The model under review builds one solid part; all positions refer to its coordinate system, in mm. A direction names the side the tool comes from. Round coordinates to 2 decimals unless told otherwise and drop trailing zeros. Loops run counter-clockwise (first coordinate to the right, second up) from the corner with the lowest first, then second, coordinate; pieces in that order, holes last. Notation, with made-up numbers: (40, -39.5) -> (70, -39.5) arc R12 cw to (70, -33.5) -> close; hole circle Ø7 at (58, 46). An arc over 180 degrees is marked (long way). Return JSON: item names as keys, results as strings. Group by question number.
```python
from build123d import *

# Parameters (mm, degrees)
SKETCH1_W           = 20.3
SKETCH1_H           = 20.5
BOSS_EXTRUDE1_DEPTH = 1.65
FILLET1_R           = 2
SKETCH2_R           = 1.25
CUT_EXTRUDE1_DEPTH  = 15.519211411
BOSS_EXTRUDE2_DEPTH = 2.65
SKETCH4_W           = 0.64
SKETCH4_H           = 0.64
BOSS_EXTRUDE3_DEPTH = 6
LPATTERN1_COUNT     = 7
LPATTERN1_PITCH     = 2.5
SKETCH5_W           = 17.5
SKETCH5_H           = 11
BOSS_EXTRUDE4_DEPTH = 1.35


with BuildPart() as part:
    # Sketch1 → Boss-Extrude1 (new body)
    with BuildSketch(Plane(origin=(0, 0, 0), x_dir=(1, 0, 0), z_dir=(0, 1, 0))):
        Rectangle(SKETCH1_W, SKETCH1_H)
    extrude(amount=BOSS_EXTRUDE1_DEPTH)

    # Fillet1
    fillet1_edges = [part.edges().sort_by_distance(p)[0] for p in [
        (10.15, 0.825, 10.25),
        (-10.15, 0.825, 10.25),
        (-10.15, 0.825, -10.25),
        (10.15, 0.825, -10.25),
    ]]
    fillet(fillet1_edges, radius=FILLET1_R)

    # Sketch2 → Cut-Extrude1 (cut, through all)
    with BuildSketch(Plane(origin=(0, 1.65, 0), x_dir=(1, 0, 0), z_dir=(0, 1, 0))):
        with Locations(Location((7.9, -8.1, 0), (0, 0, 270))):
            Circle(SKETCH2_R)
        with Locations(Location((-7.9, -8.1, 0), (0, 0, 270))):
            Circle(SKETCH2_R)
    extrude(amount=-CUT_EXTRUDE1_DEPTH, mode=Mode.SUBTRACT)

    # Sketch3 → Boss-Extrude2 (add)
    with BuildSketch(Plane(origin=(0, 1.65, 0), x_dir=(1, 0, 0), z_dir=(0, 1, 0))):
        Polygon((-8.395, 9.85), (-6.602128422, 9.85), (-6.248596673, 9.496424969), (-6.248596673, 7.703553391), (-6.602150064, 7.35), (-8.395021642, 7.35), (-8.748553391, 7.703575031), (-8.748553391, 9.496446609), align=None)
    boss_extrude2 = extrude(amount=BOSS_EXTRUDE2_DEPTH)

    # Sketch4 → Boss-Extrude3 (add)
    with BuildSketch(Plane(origin=(0, 4.3, 0), x_dir=(1, 0, 0), z_dir=(0, 1, 0))):
        with Locations((-7.498564211, 8.60001082)):
            Rectangle(SKETCH4_W, SKETCH4_H)
    boss_extrude3 = extrude(amount=BOSS_EXTRUDE3_DEPTH)

    # LPattern1: Boss-Extrude2, Boss-Extrude3 ×7
    with Locations(*[(i * LPATTERN1_PITCH, 0, 0) for i in range(1, LPATTERN1_COUNT)]):
        add(boss_extrude2)
        add(boss_extrude3)

    # Sketch5 → Boss-Extrude4 (add)
    with BuildSketch(Plane.XZ):
        with Locations((0, -1)):
            Rectangle(SKETCH5_W, SKETCH5_H)
    extrude(amount=BOSS_EXTRUDE4_DEPTH)


solid = part.part
```
1. For P1, Ø2, axis at y = 4, z = -7, coming from the +X side; P2, Ø0.7, axis at x = 5, y = 8, coming from the +Z side; P3, Ø0.5, axis at x = 5, y = 2.5, coming from the -Z side, all flat-tipped, find the tip position at first contact; note any pin that passes through.
2. We need section C-C, the plane y = 2.75. Give the number of separate pieces and of enclosed holes in the cut face, then the cut area to 3 significant figures.
3. Tool access review of faces 1 (the face through (3, 3, -7.35)), 2 (the face through (-8.749, 3, -9)), 3 (the face through (-3, 3, -9.85)), 4 (the face through (8.75, -1, -1)): name each direction out of +Z, -Z, +X, -X, +Y, -Y from which nothing blocks a thin tool from reaching the whole face with its end or side.
4. We need section A-A, the plane y = 7. Write out the cut boundary in (x, z).
5. We need section B-B, the plane z = -5. Write out the cut boundary in (x, y).
6. Wall thickness on line 1 (X direction, y = 1, z = 8.1); line 2 (Y direction, x = -2, z = -1.75); line 3 (Y direction, x = 9.25, z = 8): over which ranges is each line inside the solid? List them lowest first.
Check sheet entries:
{
 "1": {"P1": "stops at x = 8.75", "P2": "stops at z = -8.28", "P3": "stops at z = -9.85"},
 "2": {"separate pieces": "7", "enclosed holes": "0", "area": "42.0 mm²"},
 "3": {"face 1": "+Z, +X, -X, +Y", "face 2": "+Z, -Z, -X, +Y", "face 3": "-Z, +X, -X, +Y", "face 4": "+Z, -Z, +X, -Y"},
 "4": {"outline": "(-7.82, -8.92) -> (-7.18, -8.92) -> (-7.18, -8.28) -> (-7.82, -8.28) -> close; (-5.32, -8.92) -> (-4.68, -8.92) -> (-4.68, -8.28) -> (-5.32, -8.28) -> close; (-2.82, -8.92) -> (-2.18, -8.92) -> (-2.18, -8.28) -> (-2.82, -8.28) -> close; (-0.32, -8.92) -> (0.32, -8.92) -> (0.32, -8.28) -> (-0.32, -8.28) -> close; (2.18, -8.92) -> (2.82, -8.92) -> (2.82, -8.28) -> (2.18, -8.28) -> close; (4.68, -8.92) -> (5.32, -8.92) -> (5.32, -8.28) -> (4.68, -8.28) -> close; (7.18, -8.92) -> (7.82, -8.92) -> (7.82, -8.28) -> (7.18, -8.28) -> close"},
 "5": {"outline": "(-10.15, 0) -> (-8.75, 0) -> (-8.75, -1.35) -> (8.75, -1.35) -> (8.75, 0) -> (10.15, 0) -> (10.15, 1.65) -> (-10.15, 1.65) -> close"},
 "6": {"line 1": "x = -10.15 to -9.15, -6.65 to 6.65, 9.15 to 10.15", "line 2": "y = -1.35 to 1.65", "line 3": "y = 0 to 1.65"}
}
